Check sheet for the drawn part. Datum: minimum x, y, z corner. Units: mm. A direction names the side the tool comes from. Coordinates: 2 decimals unless noted, no trailing zeros. Loops run counter-clockwise (first coordinate to the right, second up) from the corner with the lowest first, then second, coordinate; pieces in that order, holes last.
Q1. Sectioned sample at B-B (y = 32). Enter the section's corners in (x, z).
Q2. Sectioned sample at D-D (x = 82). Enter the section's corners in (y, z), then the cut area to 3 significant figures.
Q3. Sectioned sample at C-C (x = 13.75). Enter the section's corners in (y, z), then the cut area to 3 significant figures.
Q4. Access from +Z, -Z, +X, -X, +Y, -Y to the whole of each face (thin tool, end or side, straight path). Record for the marked faces 4, 5 and 6.
Q5. Mould release check, pull along X, two halves, no side actions. Record for the marked faces 1, 2 and 3: +X half, -X half, draft (parallel to the pull), parting line (faces both ways), or undercut.
Q6. Material ranges on probe 1 along Z at (x, y) = (156.25, 2.9); probe 2 along Z at (x, y) = (13, 1); probe 3 along X at (y, z) = (31, 82), recorded low to high.
Q7. Go/stop test with flat-tipped pins: P1, Ø6, axis at x = 94, z = 44, coming from the -Y side; P2, Ø22, axis at x = 155.5, z = 74, coming from the +Y side; P3, Ø2, axis at y = 29.5, z = 49.5, coming from the +X side (3 decimals). Record where each tip stops, or that it passes through.
Q8. Sectioned sample at A-A (z = 70). Enter the section's corners in (x, y), then the cut area to 3 significant figures.
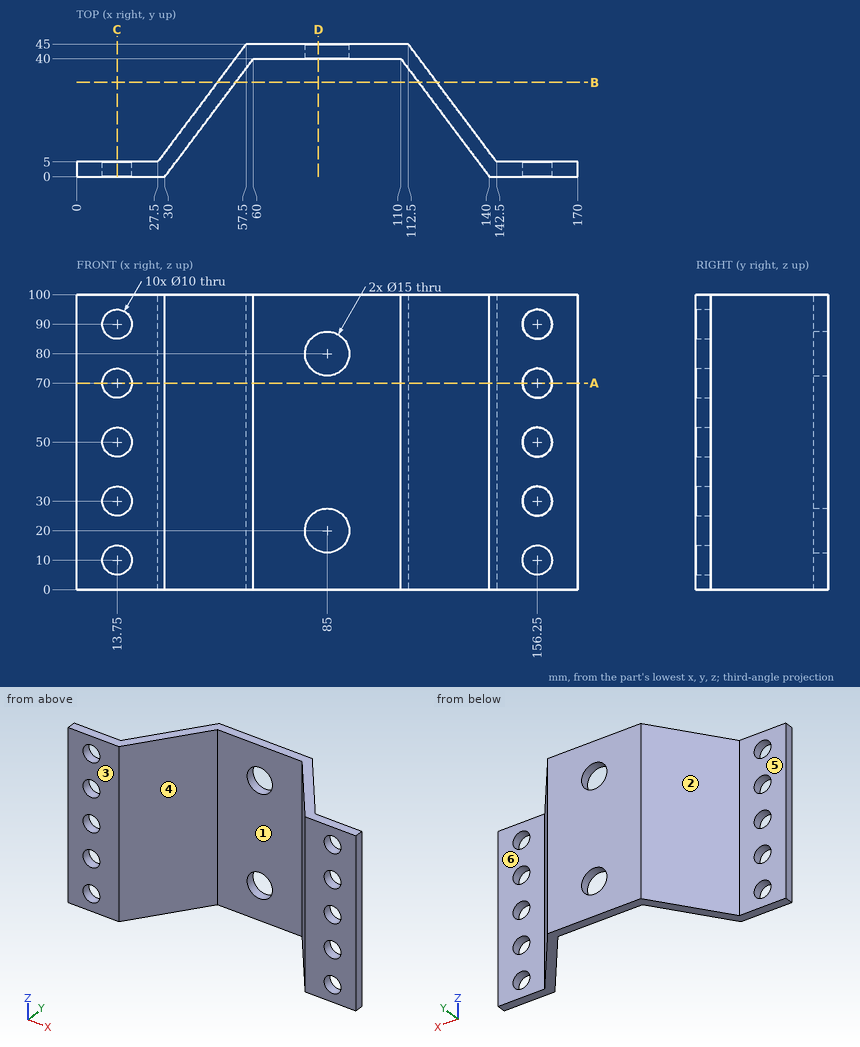
Geometry check:
1. outline: (47.75, 0) - (54, 0) - (54, 100) - (47.75, 100) - close; (116, 0) - (122.25, 0) - (122.25, 100) - (116, 100) - close
2. outline: (40, 0) - (45, 0) - (45, 13.13) - (40, 13.13) - close; (40, 26.87) - (45, 26.87) - (45, 73.13) - (40, 73.13) - close; (40, 86.87) - (45, 86.87) - (45, 100) - (40, 100) - close
2. area: 363 mm2
3. outline: (0, 0) - (5, 0) - (5, 5) - (0, 5) - close; (0, 15) - (5, 15) - (5, 25) - (0, 25) - close; (0, 35) - (5, 35) - (5, 45) - (0, 45) - close; (0, 55) - (5, 55) - (5, 65) - (0, 65) - close; (0, 75) - (5, 75) - (5, 85) - (0, 85) - close; (0, 95) - (5, 95) - (5, 100) - (0, 100) - close
3. area: 250 mm2
4. face 4: +Z, -Z, -Y
4. face 5: +Z, -Z, -X, +Y
4. face 6: +Z, -Z, +X, +Y
5. face 1: undercut
5. face 2: -X half
5. face 3: draft
6. probe 1: z = 0 to 5, 15 to 25, 35 to 45, 55 to 65, 75 to 85, 95 to 100
6. probe 2: z = 0 to 5.06, 14.94 to 25.06, 34.94 to 45.06, 54.94 to 65.06, 74.94 to 85.06, 94.94 to 100
6. probe 3: x = 47 to 53.25, 116.75 to 123
7. P1: stops at y = 40
7. P2: stops at y = 5
7. P3: stops at x = 124.875
8. outline: (0, 0) - (8.75, 0) - (8.75, 5) - (0, 5) - close; (18.75, 0) - (30, 0) - (60, 40) - (110, 40) - (140, 0) - (151.25, 0) - (151.25, 5) - (142.5, 5) - (112.5, 45) - (57.5, 45) - (27.5, 5) - (18.75, 5) - close; (161.25, 0) - (170, 0) - (170, 5) - (161.25, 5) - close
8. area: 950 mm2
